```python
from build123d import *

# Parameters (mm, degrees)
F0_W     = 101.6
F0_H     = 101.6
F1_DEPTH = 3.175
F1_TAPER = 3
F2_T     = -14.0335
F4_ANGLE = 45


# Not quite as in the source:
# - a feature of the source that left no trace in its solid (it failed there, or was rolled back) is left out


with BuildPart() as f1:
    # F0 (on Top) → F1 (new body)
    with BuildSketch(Plane.XY):
        Rectangle(F0_W, F0_H)
    extrude(amount=F1_DEPTH, taper=F1_TAPER)

    # F2
    f2_openings = [f1.faces().sort_by_distance(p)[0] for p in [
        (0, 0, 3.175),
        (0, 0, 0),
    ]]
    offset(amount=F2_T, openings=f2_openings)


with BuildPart() as f1_1:
    # F4: moved
    add(f1.part.rotate(Axis((0, 0, 69.4056898355), (0, 0, 1)), F4_ANGLE))


solid = f1_1.part
```
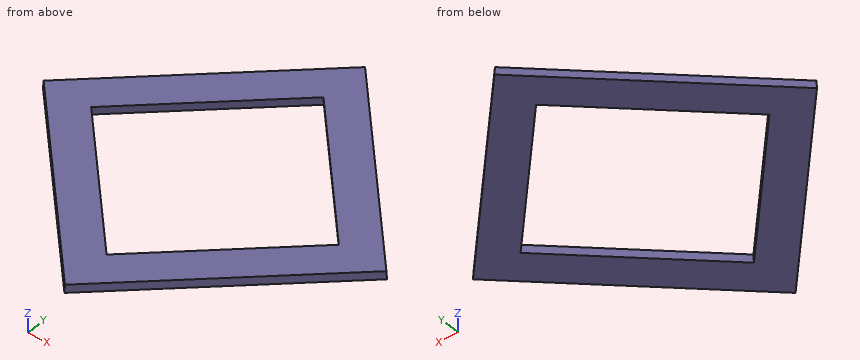
The listing builds one solid part. Answer for the finished solid, in the listing's coordinates (mm). Coordinates: 2 decimals unless noted, no trailing zeros. Loops run counter-clockwise (first coordinate to the right, second up) from the corner with the lowest first, then second, coordinate; pieces in that order, holes last. Notation, with made-up numbers: (-22, 32.5) -> (31, 32.5) arc R17 ccw to (31, 51.5) -> close; hole circle Ø4 at (43.5, 34). An arc over 180 degrees is marked (long way). Return JSON: item names as keys, results as strings. Group by question number.
(1) A cutting plane is placed at D-D on x = -59.5. Write down the section's boundary in (y, z) (3 decimals).
(2) Find the intervals of material crossed by probe 1 along X at (y, z) = (-17.5, 0.9); probe 2 along Y at (x, z) = (-35, 3); probe 3 along X at (y, z) = (-44, 1.95), in increasing order. Write a range as from..to.
(3) A cutting plane is placed at B-B on x = -30. Write down the section's boundary in (y, z) (3 decimals).
(4) A cutting plane is placed at A-A on z = 1.65. Write down the section's boundary in (x, y), and give its area (3 significant figures).
(5) A cutting plane is placed at C-C on y = 6.5. Write down the section's boundary in (x, z) (3 decimals), and give its area (3 significant figures).
The answers:
{
 "1": {"outline": "(-12.342, 0) -> (12.342, 0) -> (12.107, 3.175) -> (-12.107, 3.175) -> close"},
 "2": {"probe 1": "x = -54.28..-34.4, 34.4..54.28", "probe 2": "y = -36.62..-16.75, 16.75..36.62", "probe 3": "x = -27.7..-7.82, 7.82..27.7"},
 "3": {"outline": "(-41.842, 0) -> (-21.968, 0) -> (-21.733, 3.175) -> (-41.607, 3.175) -> close; (21.733, 3.175) -> (21.968, 0) -> (41.842, 0) -> (41.607, 3.175) -> close"},
 "4": {"outline": "(-71.72, 0) -> (0, -71.72) -> (71.72, 0) -> (0, 71.72) -> close; hole (-51.85, 0) -> (0, -51.85) -> (51.85, 0) -> (0, 51.85) -> close", "area": "4,910 mm^2"},
 "5": {"outline": "(-65.342, 0) -> (-45.468, 0) -> (-45.233, 3.175) -> (-65.107, 3.175) -> close; (45.233, 3.175) -> (45.468, 0) -> (65.342, 0) -> (65.107, 3.175) -> close", "area": "126 mm^2"}
}
